from build123d import *

# Parameters (mm, degrees)
F0_W     = 92.075
F0_H     = 250.825
F1_DEPTH = 9.525
F3_D     = 6.7564
F5_D     = 5
F5_DEPTH = 28.4
F5_TIP   = 1.5021515476


# Not quite as in the source:
# - a feature names something its author has since deleted; it is built from what else it names


with BuildPart() as f1:
    # F0 (on Front) → F1 (new body)
    with BuildSketch(Plane.XZ):
        with Locations((46.0375, 125.4125)):
            Rectangle(F0_W, F0_H)
    extrude(amount=-F1_DEPTH)

    # F3 (through all)
    with Locations(Plane.XZ):
        with Locations((46.0375, 241.3), (84.1375, 241.3), (7.9375, 241.3)):
            Hole(F3_D / 2)

    # F5
    with Locations(Plane(origin=(0, 0, 0), x_dir=(1, 0, 0), z_dir=(0, 0, -1))):
        with Locations((7.9375, -4.7625), (33.3375, -4.7625), (58.7375, -4.7625), (84.1375, -4.7625), (109.5375, -4.7625), (134.9375, -4.7625)):
            Hole(F5_D / 2, depth=F5_DEPTH)
            with Locations((0, 0, -(F5_DEPTH + F5_TIP / 2))):  # 118° drill point
                Cone(0, F5_D / 2, F5_TIP, mode=Mode.SUBTRACT)


solid = f1.part
Input: part model. Units: mm. Frame: model coordinates. A direction names the side the tool comes from. Give positions to 0.01 mm unless a question says otherwise; leave off trailing zeros. Loops run counter-clockwise (first coordinate to the right, second up) from the corner with the lowest first, then second, coordinate; pieces in that order, holes last. Notation, with made-up numbers: (84, 35.25) -> (103, 35.25) arc R24 ccw to (103, 47.25) -> close; hole circle Ø6 at (17.5, -17). An arc over 180 degrees is marked (long way). Answer as a JSON object with one key per item and string values. Group by question number.
Item 1: Line query: probe 1 along X at (y, z) = (5.75, 241.3) (3 decimals); probe 2 along X at (y, z) = (8, 239) (3 decimals); probe 3 along Z at (x, y) = (57, 4.75) (3 decimals). Output: solid intervals per line, ascending.
Item 2: Pin query (flat end, axial travel): P1, Ø9, axis at x = 46.04, z = 241.3, coming from the +Y side (3 decimals); P2, Ø6, axis at x = 84.14, z = 241.3, coming from the +Y side; P3, Ø4.5, axis at x = 58.74, y = 4.76, coming from the -Z side. Return the tip coordinate at first contact, or that it passes through.
Item 3: Reachability of faces 4 (the cylindrical face through (61.235, 4.653, 14.399)), 5 (the flat face through (92.075, 5, 124)) from +Z, -Z, +X, -X, +Y, -Y: full face, straight path, thin tool, end or side. Return the list, or none.
Item 4: Cut plane B-B, the plane x = 45.5. Return the cut outline in (y, z) (3 decimals), and give its area (3 significant figures).
Item 5: Pull-direction query (X, two-part tool) for faces 1 (the flat face through (0, 5, 124)), 2 (the flat face through (45, 5, 250.825)), 3 (the cylindrical face through (10.435, 4.653, 14.399)); classes: released by +X, released by -X, zero draft, split by the parting line, or undercut.
Item 6: Cut plane A-A, the plane z = 241.3. Return the cut outline in (x, y) (3 decimals), and give its area (3 significant figures).
Checks:
{
 "1": {"probe 1": "x = 0 to 4.559, 11.316 to 42.659, 49.416 to 80.759, 87.516 to 92.075", "probe 2": "x = 0 to 5.463, 10.412 to 43.563, 48.512 to 81.663, 86.612 to 92.075", "probe 3": "z = 28.858 to 250.825"},
 "2": {"P1": "stops at y = 9.525", "P2": "passes through", "P3": "stops at z = 28.55"},
 "3": {"face 4": "-Z", "face 5": "+Z, -Z, +X, +Y, -Y"},
 "4": {"outline": "(0, 0) -> (9.525, 0) -> (9.525, 237.965) -> (0, 237.965) -> close; (0, 244.635) -> (9.525, 244.635) -> (9.525, 250.825) -> (0, 250.825) -> close", "area": "2,330 mm²"},
 "5": {"face 1": "released by -X", "face 2": "zero draft", "face 3": "undercut"},
 "6": {"outline": "(0, 0) -> (4.559, 0) -> (4.559, 9.525) -> (0, 9.525) -> close; (11.316, 0) -> (42.659, 0) -> (42.659, 9.525) -> (11.316, 9.525) -> close; (49.416, 0) -> (80.759, 0) -> (80.759, 9.525) -> (49.416, 9.525) -> close; (87.516, 0) -> (92.075, 0) -> (92.075, 9.525) -> (87.516, 9.525) -> close", "area": "684 mm²"}
}
